from build123d import *

# Parameters (mm, degrees)
SKETCH1_R           = 25
BOSS_EXTRUDE1_DEPTH = 40
CUT_EXTRUDE1_REACH  = 100.995
SKETCH2_R           = 11
CUT_EXTRUDE3_REACH  = 100.995


with BuildPart() as part:
    # Sketch1 → Boss-Extrude1 (new body)
    with BuildSketch(Plane.XY):
        Polygon((25, 0), (-25, 0), (-14, -11), (-40, -11), (-40, 49), (-10, 79), (0, 79), (10, 79), (40, 49), (40, -11), (14, -11), align=None)
        with Locations((0, 39)):
            Circle(SKETCH1_R, mode=Mode.SUBTRACT)
    extrude(amount=-BOSS_EXTRUDE1_DEPTH)

    # Sketch2 → Cut-Extrude1 (cut, up to next)
    with BuildSketch(Plane(origin=(44.5, 44.5, 0), x_dir=(0, 0, -1), z_dir=(0.707106781, 0.707106781, 0)), mode=Mode.PRIVATE) as cut_extrude1_sk1:
        with Locations((20, 27.790367902)):
            Circle(SKETCH2_R)
    cut_extrude1_tool1 = extrude(cut_extrude1_sk1.sketch, amount=-CUT_EXTRUDE1_REACH, mode=Mode.PRIVATE) & part.part
    add(cut_extrude1_tool1.solids().sort_by_distance((24.849242, 64.150758, -20))[0], mode=Mode.SUBTRACT)

    # Sketch3 → Cut-Extrude3 (cut, up to next)
    with BuildSketch(Plane(origin=(-44.5, 44.5, 0), x_dir=(0, 0, 1), z_dir=(-0.707106781, 0.707106781, 0)), mode=Mode.PRIVATE) as cut_extrude3_sk1:
        Polygon((-8.452994616, 27.790367902), (-14.226497308, 37.790367902), (-25.773502692, 37.790367902), (-31.547005384, 27.790367902), (-25.773502692, 17.790367902), (-14.226497308, 17.790367902), align=None)
    cut_extrude3_tool1 = extrude(cut_extrude3_sk1.sketch, amount=-CUT_EXTRUDE3_REACH, mode=Mode.PRIVATE) & part.part
    add(cut_extrude3_tool1.solids().sort_by_distance((-24.849242, 64.150758, -20))[0], mode=Mode.SUBTRACT)


solid = part.part
CAD build for the part. Positions are in the model's coordinates, mm. A direction names the side the tool comes from. Give positions to 0.01 mm unless a question says otherwise; leave off trailing zeros. Order: outer loops, then holes, each group sorted by start corner. A loop starts at its lowest first (then second) coordinate and runs counter-clockwise, first axis right, second up. Notation, with made-up numbers: (0.5, 0.5) - (28.5, 0.5) arc R17 ccw to (28.5, 20.5) - close; hole circle Ø11 at (-25.75, 82.25). An arc over 180 degrees is marked (long way). Write each question's results on one line, items separated by ' | '.
1. Saw through at A-A on y = 39. List the corners of the cut face in (x, z).
Calculated:
outline: (-40, -40) - (-25, -40) - (-25, 0) - (-40, 0) - close; (25, -40) - (40, -40) - (40, 0) - (25, 0) - close
2. Pull direction X, two halves, no side cores. Call faces 1 (the face through (31, 58, -11)), 2 (the face through (-5.42, 14.594, -19.72)), 3 (the face through (27, -11, -20)), 4 (the face through (-20, -5, -20)): released by +X, released by -X, zero draft, split by the parting line, or undercut.
Calculated:
face 1: released by +X | face 2: undercut | face 3: zero draft | face 4: undercut
3. Probe L1, parallel to Y at x = 0, z = -22; L2, parallel to Y at x = -17, z = -5; L3, parallel to X at y = 56.5, z = -37. List the from-to ranges inside material, lowest first. Write a range as from..to.
Calculated:
L1: y = 0..14, 64..79 | L2: y = -11..-8, 0..20.67, 57.33..72 | L3: x = -32.5..-17.85, 17.85..32.5
4. Pin check, flat tips, straight feed: pin 1 (1 mm diameter, centred on y = 58.5, z = -22.5, fed in from -X); pin 2 (3 mm diameter, centred on x = 4, z = -20, fed in from -Y). Stop position of each tip, or through.
Calculated:
pin 1: passes through | pin 2: stops at y = 0
5. Saw through at D-D on x = 22. Count the separate pieces of the cut face and the enclosed holes in it, and give its area (3 significant figures).
Calculated:
separate pieces: 4 | enclosed holes: 0 | area: 1,720 mm2
6. 3-axis set-ups, long thin cutter, end or side, ignore diameter. For faces 5 (the face through (-16.894, 63.365, -28.62)), 6 (the face through (-27.61, 52.77, -20.08)), 7 (the face through (0, 0, -20)): which of +Z, -Z, +X, -X, +Y, -Y reach the whole face in a straight line?
Calculated:
face 5: none | face 6: +Y | face 7: +Z, -Z
7. Saw through at B-B on x = 0. List the corners of the cut face in (y, z), and give its area (3 significant figures).
Calculated:
outline: (0, -40) - (14, -40) - (14, 0) - (0, 0) - close; (64, -40) - (79, -40) - (79, 0) - (64, 0) - close | area: 1,160 mm2
8. Saw through at C-C on z = -27. List the corners of the cut face in (x, y).
Calculated:
outline: (-40, -11) - (-14, -11) - (-25, 0) - (25, 0) - (14, -11) - (40, -11) - (40, 49) - (30.85, 58.15) - (22.53, 49.83) arc R25 cw (long way) to (-22.25, 50.41) - (-30.42, 58.58) - (-40, 49) - close; (-19.28, 69.72) - (-11.01, 61.45) arc R25 cw to (10.42, 61.72) - (18.85, 70.15) - (10, 79) - (-10, 79) - close
